```python
from build123d import *

# Parameters (mm, degrees)
SKETCH1_R            = 1.7859375
BOSS_EXTRUDE1_DEPTH  = 1.5875
FILLET1_R            = 3.175
FILLET1_OF_MIRROR1_R = 3.175


with BuildPart() as part:
    # Sketch1 → Boss-Extrude1 (new body)
    with BuildSketch(Plane.XY):
        with BuildLine():
            Line((-8.73125, 0), (0, 0))
            Line((0, 0), (0, 5.55625))
            Line((0, 5.55625), (-7.552307909, 5.55625))
            ThreePointArc((-7.552307909, 5.55625), (-9.862459716, 6.553217945), (-10.721810073, 8.918014642))
            ThreePointArc((-10.721810073, 8.918014642), (-14.966353253, 12.634896917), (-17.517188185, 7.602541425))
            ThreePointArc((-17.517188185, 7.602541425), (-17.263166539, 5.68441597), (-18.169650628, 3.9750246))
            ThreePointArc((-18.169650628, 3.9750246), (-16.444084642, -5.120650031), (-8.73125, 0))
        make_face()
        with Locations((-14.2875, 0)):
            Circle(SKETCH1_R, mode=Mode.SUBTRACT)
        with Locations((-14.2875, 9.128125)):
            Circle(SKETCH1_R, mode=Mode.SUBTRACT)
    boss_extrude1 = extrude(amount=BOSS_EXTRUDE1_DEPTH)

    # Fillet1
    fillet1_edges = [part.edges().sort_by_distance(p)[0] for p in [
        (-8.73125, 0, 0.79375),
    ]]
    fillet(fillet1_edges, radius=FILLET1_R)

    # Mirror1: Boss-Extrude1 across plane
    add(boss_extrude1.mirror(Plane(origin=(0, 0, 1.5875), x_dir=(0, 0, 1), z_dir=(1, 0, 0))))

    # Fillet1 of Mirror1
    fillet1_of_mirror1_edges = [part.edges().sort_by_distance(p)[0] for p in [
        (8.73125, 0, 0.79375),
    ]]
    fillet(fillet1_of_mirror1_edges, radius=FILLET1_OF_MIRROR1_R)


solid = part.part
```
Source: CAD feature listing. Evaluate the final solid. Frame: model axes, mm. A direction names the side the tool comes from. Round coordinates to 2 decimals unless told otherwise and drop trailing zeros. Loops run counter-clockwise (first coordinate to the right, second up) from the corner with the lowest first, then second, coordinate; pieces in that order, holes last. Notation, with made-up numbers: M -39,79.5 L -35,79.5 A26 cw -35,106.5 Z; hole C 81,31.5 d3. An arc over 180 degrees is marked long. Put each result on its own line as item: value.
(1) First-contact query: pin 1 (3 mm diameter, centred on x = 14.29, y = 0, fed in from -Z); pin 2 (0.5 mm diameter, centred on x = -2.5, z = 0.5, fed in from +Y). Flat tips, straight axial feed; report the tip coordinate or a pass-through.
Solutions:
pin 1: through
pin 2: y = 5.56
(2) Ray query, line 1 (X direction, y = 9, z = 0.4); line 2 (X direction, y = 10, z = 0.4); line 3 (Y direction, x = 13, z = 0.2). Return the intervals inside material, ascending. Write a range as [from, to].
Solutions:
line 1: [-17.86, -16.07], [-12.51, -10.72], [10.72, 12.51], [16.07, 17.86]
line 2: [-17.75, -15.85], [-12.73, -10.82], [10.82, 12.73], [15.85, 17.75]
line 3: [-5.41, -1.24], [1.24, 7.89], [10.37, 12.46]
(3) Pull-direction query (X, two-part tool) for faces 4 (the face through (-17.26, 5.71, 0.78)), 5 (the face through (0, 2, 0)), 6 (the face through (17.26, 5.71, 0.78)), 7 (the face through (-7.923, -0.538, 0.805)); classes: released by +X, released by -X, zero draft, split by the parting line, or undercut.
Solutions:
face 4: released by -X
face 5: zero draft
face 6: released by +X
face 7: undercut
(4) Access query for faces 1 (the face through (7.923, -0.538, 0.805)), 2 (the face through (0, 5.556, 1)), 3 (the face through (17.469, -4.555, 0.783)). Directions: +Z, -Z, +X, -X, +Y, -Y. A direction counts if a zero-diameter tool reaches every point of the face in a straight line with its end or side. Return the directions, or none.
Solutions:
face 1: +Z, -Z, -Y
face 2: +Z, -Z, +Y
face 3: +Z, -Z
(5) Section C-C, the plane z = 1. State how many separate pieces and enclosed holes the cut face has, and give its area (3 significant figures).
Solutions:
separate pieces: 1
enclosed holes: 4
area: 361 mm²
(6) Section A-A, the plane y = 11.75. Return loops of the section in (x, z), and give its area (3 significant figures).
Solutions:
outline: M -16.71,0 L -11.86,0 L -11.86,1.59 L -16.71,1.59 Z; M 11.86,0 L 16.71,0 L 16.71,1.59 L 11.86,1.59 Z
area: 15.4 mm²
(7) Section D-D, the plane x = 3.5. Return loops of the section in (y, z), and give its area (3 significant figures).
Solutions:
outline: M 0,0 L 5.56,0 L 5.56,1.59 L 0,1.59 Z
area: 8.82 mm²
(8) Section B-B, the plane y = 1.25. Return loops of the section in (x, z), and give its area (3 significant figures).
Solutions:
outline: M -19.7,0 L -15.56,0 L -15.56,1.59 L -19.7,1.59 Z; M -13.01,0 L 13.01,0 L 13.01,1.59 L -13.01,1.59 Z; M 15.56,0 L 19.7,0 L 19.7,1.59 L 15.56,1.59 Z
area: 54.5 mm²
